from build123d import *

# Parameters (mm, degrees)
F0_W     = 25.4
F0_H     = 38.1
F1_DEPTH = 12.7
F2_R     = 6.5370938685
F3_DEPTH = 12.701
F4_W     = 12.7907153219
F4_H     = 10.0692855194
F5_DEPTH = 19.05
F6_W     = 13.0628570914
F6_H     = 28.0307149515
F7_DEPTH = 25.4


with BuildPart() as f1:
    # F0 (on Top) → F1 (new body)
    with BuildSketch(Plane.XY):
        Rectangle(F0_W, F0_H)
        with BuildLine():
            ThreePointArc((12.7, -19.05), (31.75, 0), (12.7, 19.05))
            Line((12.7, 19.05), (12.7, -19.05))
        make_face()
    extrude(amount=F1_DEPTH)

    # F2 (on Top) → F3 (cut, through all)
    with BuildSketch(Plane.XY):
        with Locations((16.3285713643, 0)):
            Circle(F2_R)
    extrude(amount=F3_DEPTH, mode=Mode.SUBTRACT)

    # F4 (on Top) → F5 (join)
    with BuildSketch(Plane.XY):
        with Locations((-6.3953576609, -14.0153574757)):
            Rectangle(F4_W, F4_H)
    extrude(amount=F5_DEPTH)

    # F6 (on Top) → F7 (join)
    with BuildSketch(Plane.XY):
        with Locations((-6.5314285457, 5.0346427597)):
            Rectangle(F6_W, F6_H)
    extrude(amount=F7_DEPTH)


solid = f1.part
Verification items for the finished model (mm, model axes). A direction names the side the tool comes from. Coordinates: 2 decimals unless noted, no trailing zeros. Write each loop counter-clockwise with the first axis right and the second up, starting at its lowest first coordinate (ties: lowest second). Pieces come first, ordered by that corner, then holes. Notation, with made-up numbers: M 40,66 L 69,66 A29 cw 69,104 Z; hole C -2.5,-25 d4. An arc over 180 degrees is marked long. One line per question, with ' | ' between items.
1) Depth check by flat-ended pin: pin 1 Ø4 at (x, z) = (16.5, 12) entering from +Y; pin 2 Ø5 at (x, y) = (-9, -12) entering from +Z; pin 3 Ø6.5 at (y, z) = (-5, 16) entering from +X. Enter the tip coordinate at first touch or a pass-through.
Solutions:
pin 1: y = 18.96 | pin 2: z = 19.05 | pin 3: x = 0
2) Access from +Z, -Z, +X, -X, +Y, -Y to the whole of each face (thin tool, end or side, straight path). Record for faces 4 (the face through (-6, -14, 19.05)), 5 (the face through (-12.791, -14, 9)), 6 (the face through (9, 0, 12.7)).
Solutions:
face 4: +Z, +X, -X, -Y | face 5: +Z, -Z, -X, -Y | face 6: +Z, +X, +Y, -Y
3) Release check for a two-part mould opening along Y. For faces 1 (the face through (31.745, -0.419, 6.261)), 2 (the face through (-13.063, 5, 13)), 3 (the face through (22.564, 1.964, 6.261)) record: +Y half, -Y half, draft (parallel to the pull), parting line (faces both ways), or undercut.
Solutions:
face 1: parting line | face 2: draft | face 3: undercut
4) Sectioned sample at D-D on z = 13.75. Record the cut outline in (x, y), then the cut area to 3 significant figures.
Solutions:
outline: M -13.06,-8.98 L -12.79,-8.98 L -12.79,-19.05 L 0,-19.05 L 0,19.05 L -13.06,19.05 Z | area: 495 mm^2
5) Sectioned sample at A-A on y = 0. Record the cut outline in (x, z), then the cut area to 3 significant figures.
Solutions:
outline: M -13.06,0 L 9.79,0 L 9.79,12.7 L 0,12.7 L 0,25.4 L -13.06,25.4 Z; M 22.87,0 L 31.75,0 L 31.75,12.7 L 22.87,12.7 Z | area: 569 mm^2
6) Material ranges on L1, parallel to X at y = 0, z = 5.75; L2, parallel to Z at x = 4.5, y = 9; L3, parallel to Y at x = -2, z = 22.25, recorded low to high.
Solutions:
L1: -13.06 to 9.79, 22.87 to 31.75 | L2: 0 to 12.7 | L3: -8.98 to 19.05
7) Sectioned sample at C-C on x = -2. Record the cut outline in (y, z).
Solutions:
outline: M -19.05,0 L 19.05,0 L 19.05,25.4 L -8.98,25.4 L -8.98,19.05 L -19.05,19.05 Z
8) Sectioned sample at B-B on z = 3.75. Record the cut outline in (x, y), then the cut area to 3 significant figures.
Solutions:
outline: M -13.06,-8.98 L -12.79,-8.98 L -12.79,-19.05 L 12.7,-19.05 A19.05 ccw 12.7,19.05 L -13.06,19.05 Z; hole C 16.33,0 d13.07 | area: 1,410 mm^2
